Geometry check sheet. Reference: the model listing, model coordinates, mm. Face numbers are marked on the shaded views. A direction names the side the tool comes from. Give positions to 0.01 mm unless a question says otherwise; leave off trailing zeros. Order: outer loops, then holes, each group sorted by start corner. A loop starts at its lowest first (then second) coordinate and runs counter-clockwise, first axis right, second up. Notation, with made-up numbers: M 20,2 L 44,2 A23 ccw 44,35 Z; hole C -30.5,24 d8. An arc over 180 degrees is marked long. Answer as CSV lines item,"result".
from build123d import *

# Parameters (mm, degrees)
SKETCH1_W           = 15
SKETCH1_H           = 15
BOSS_EXTRUDE1_DEPTH = 3
SKETCH2_W           = 3
SKETCH2_H           = 15
BOSS_EXTRUDE2_DEPTH = 12
SKETCH3_R           = 2
CUT_EXTRUDE1_DEPTH  = 12
SKETCH4_R           = 2
CUT_EXTRUDE2_DEPTH  = 12


with BuildPart() as part:
    # Sketch1 → Boss-Extrude1 (new body)
    with BuildSketch(Plane.XY):
        Rectangle(SKETCH1_W, SKETCH1_H)
    extrude(amount=BOSS_EXTRUDE1_DEPTH)

    # Sketch2 → Boss-Extrude2 (add)
    with BuildSketch(Plane.XY.offset(3)):
        with Locations((-6, 0)):
            Rectangle(SKETCH2_W, SKETCH2_H)
    extrude(amount=BOSS_EXTRUDE2_DEPTH)

    # Sketch3 → Cut-Extrude1 (cut)
    with BuildSketch(Plane(origin=(0, 0, 0), x_dir=(-1, 0, 0), z_dir=(0, 0, -1))):
        with Locations((-1.5, 0)):
            Circle(SKETCH3_R)
    extrude(amount=-CUT_EXTRUDE1_DEPTH, mode=Mode.SUBTRACT)

    # Sketch4 → Cut-Extrude2 (cut)
    with BuildSketch(Plane.ZY.offset(7.5)):
        with Locations(Location((9, 0, 0), (0, 0, 270))):
            Circle(SKETCH4_R)
    extrude(amount=-CUT_EXTRUDE2_DEPTH, mode=Mode.SUBTRACT)


solid = part.part
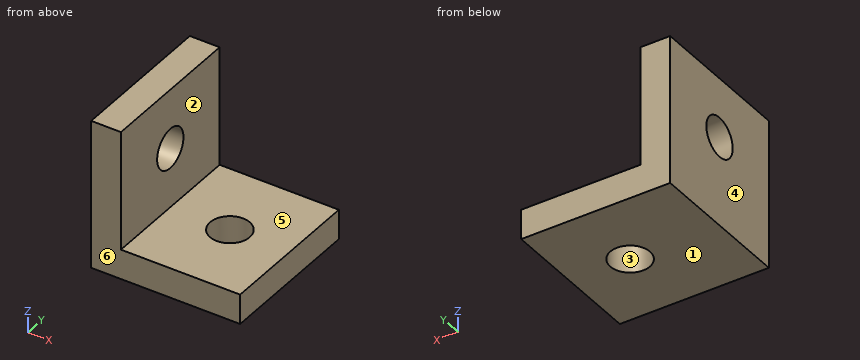
(1) Gauge pin test, flat end, axial feed: P1, Ø1.5, axis at y = 5, z = 6.5, coming from the +X side. Record the tip position at first contact, or that the pin passes through.
The answers:
P1,"stops at x = -4.5"
(2) Draft check along X on the marked faces 1, 2, 3 and 4. Enter one of: +X half, -X half, draft (parallel to the pull), parting line (faces both ways), or undercut.
The answers:
face 1,"draft"
face 2,"+X half"
face 3,"undercut"
face 4,"-X half"
(3) Material ranges on line 1 (Z direction, x = -5.3, y = 0); line 2 (Y direction, x = 1.5, z = 1.75); line 3 (X direction, y = -2, z = 13.25), recorded low to high.
The answers:
line 1,"z = 0 to 7, 11 to 15"
line 2,"y = -7.5 to -2, 2 to 7.5"
line 3,"x = -7.5 to -4.5"
(4) Section check C-C on z = 9. Enter the section's corners in (x, y).
The answers:
outline,"M -7.5,-7.5 L -4.5,-7.5 L -4.5,-2 L -7.5,-2 Z; M -7.5,2 L -4.5,2 L -4.5,7.5 L -7.5,7.5 Z"
(5) Section check D-D on y = -3.5. Enter the section's corners in (x, z).
The answers:
outline,"M -7.5,0 L 7.5,0 L 7.5,3 L -4.5,3 L -4.5,15 L -7.5,15 Z"
(6) Section check A-A on y = 0. Enter the section's corners in (x, z).
The answers:
outline,"M -7.5,0 L -0.5,0 L -0.5,3 L -4.5,3 L -4.5,7 L -7.5,7 Z; M -7.5,11 L -4.5,11 L -4.5,15 L -7.5,15 Z; M 3.5,0 L 7.5,0 L 7.5,3 L 3.5,3 Z"
(7) Section check B-B on x = 1.5. Enter the section's corners in (y, z).
The answers:
outline,"M -7.5,0 L -2,0 L -2,3 L -7.5,3 Z; M 2,0 L 7.5,0 L 7.5,3 L 2,3 Z"
(8) Tool access check on the marked faces 5 and 6. Record the directions out of +Z, -Z, +X, -X, +Y, -Y that give a thin tool (end or side, any length) a straight path to the whole face; none if there is none.
The answers:
face 5,"+Z, +X, +Y, -Y"
face 6,"+Z, -Z, +X, -X, -Y"
